The model under review builds one solid part; all positions refer to its coordinate system, in mm. Face numbers are marked on the shaded views. A direction names the side the tool comes from. Give positions to 0.01 mm unless a question says otherwise; leave off trailing zeros. Order: outer loops, then holes, each group sorted by start corner. A loop starts at its lowest first (then second) coordinate and runs counter-clockwise, first axis right, second up. Notation, with made-up numbers: (-27.75, 47.5) -> (5.25, 47.5) arc R7 ccw to (5.25, 54.5) -> close; hole circle Ø1 at (55.5, 69). An arc over 180 degrees is marked (long way). Answer as a JSON object with one key per item and string values. Group by question number.
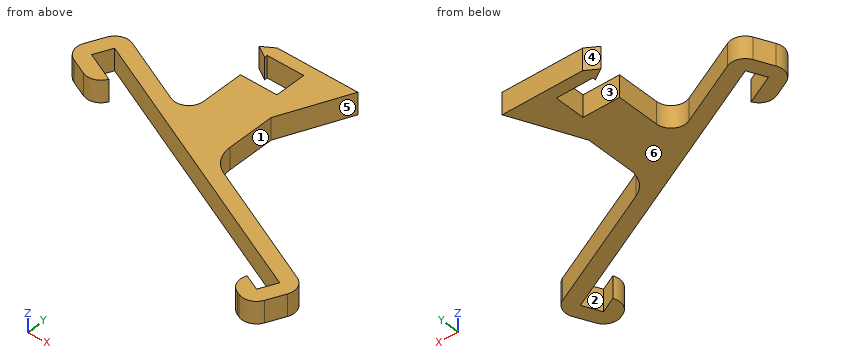
from build123d import *

# Parameters (mm, degrees)
BOSS_EXTRUDE1_DEPTH = 15
FILLET1_R           = 10
FILLET2_R           = 20


with BuildPart() as part:
    # Sketch1 → Boss-Extrude1 (new body)
    with BuildSketch(Plane.XY):
        Polygon((0, 0), (-25, 0), (-25, -2), (-33, 2.914001084), (-25, 8), (10, 8), (30, 8), (10, -37), (10, -82), (115.477706991, -131.185062534), (101.531304353, -161.093219507), (81.592533038, -151.795617748), (85.818715656, -142.732539878), (96.6944091, -147.803959019), (102.188446503, -136.021957787), (-88.136188775, -47.272122822), (-93.630226177, -59.054124053), (-73.691454863, -68.351725812), (-77.91763748, -77.414803682), (-106.919486665, -63.891019306), (-92.973084028, -33.982862334), (-25, -65.679231965), (-25, -21), (0, -21), align=None)
    extrude(amount=BOSS_EXTRUDE1_DEPTH)

    # Fillet1
    fillet1_edges = [part.edges().sort_by_distance(p)[0] for p in [
        (115.477706991, -131.185062534, 7.5),
        (101.531304353, -161.093219507, 7.5),
        (81.592533038, -151.795617748, 7.5),
        (-77.91763748, -77.414803682, 7.5),
        (-106.919486665, -63.891019306, 7.5),
        (-92.973084028, -33.982862334, 7.5),
        (-25, -65.679231965, 7.5),
    ]]
    fillet(fillet1_edges, radius=FILLET1_R - 0.0001)  # a hair under: the kernel refuses the full size

    # Fillet2
    fillet2_edges = [part.edges().sort_by_distance(p)[0] for p in [
        (10, -82, 7.5),
    ]]
    fillet(fillet2_edges, radius=FILLET2_R)


solid = part.part
1. Take a section at D-D on x = -71.5. Give the boundary of the cut face in (y, z), plus the area to 3 significant figures.
2. For probe 1 along X at (y, z) = (-56, 1.5); probe 2 along Y at (x, z) = (23, 13.5); probe 3 along X at (y, z) = (-51, 4.25), list the stretches that pass through material, from the lowest coordinate up. Write a range as [from, to].
3. Take a section at B-B on x = -3. Give the boundary of the cut face in (y, z).
4. Take a section at C-C on y = -116.5. Give the boundary of the cut face in (x, z), plus the area to 3 significant figures.
5. Draft analysis for pull direction Y (two halves, no side actions). For the marked faces 4, 5 and 6, state which applies: pulls with the +Y half, pulls with the -Y half, needs draft (parallel to the pull), parting line crosses it, or undercut.
6. Machinability: for the marked faces 1, 2 and 3, which of the approach directions +Z, -Z, +X, -X, +Y, -Y give a long, thin tool a straight path to every point of the face, cutting with its end or side? Answer none if there is none.
7. For pin 1 (5 mm diameter, centred on y = -23.5, z = 9.5, fed in from -X); pin 2 (4.5 mm diameter, centred on y = -37.5, z = 7, fed in from -X); pin 3 (7.5 mm diameter, centred on x = -13.5, z = 11, fed in from -Y); pin 4 (2 mm diameter, centred on x = 67.5, y = -123, fed in from -Z), all flat-tipped, find the tip position at first contact; note any pin that passes through.
Checks:
{
 "1": {"outline": "(-55.03, 0) -> (-44, 0) -> (-44, 15) -> (-55.03, 15) -> close", "area": "166 mm2"},
 "2": {"probe 1": "x = [-103.15, -92.21], [-69.42, -45.76], [-27.01, 10]", "probe 2": "y = [-99.1, -88.06], [-7.75, 8]", "probe 3": "x = [-100.91, -89.87], [-80.14, -56.48], [-25.05, 10]"},
 "3": {"outline": "(-86.97, 0) -> (-21, 0) -> (-21, 15) -> (-86.97, 15) -> close; (0, 0) -> (8, 0) -> (8, 15) -> (0, 15) -> close"},
 "4": {"outline": "(60.32, 0) -> (83.99, 0) -> (83.99, 15) -> (60.32, 15) -> close", "area": "355 mm2"},
 "5": {"face 4": "pulls with the +Y half", "face 5": "undercut", "face 6": "needs draft"},
 "6": {"face 1": "+Z, -Z, +X", "face 2": "+Z, -Z", "face 3": "+Z, -Z, -X"},
 "7": {"pin 1": "stops at x = -25", "pin 2": "stops at x = -94.73", "pin 3": "stops at y = -83.82", "pin 4": "passes through"}
}
